Check sheet for the modelled part. Datum: model origin and axes. Units: mm. Give positions to 0.01 mm unless a question says otherwise; leave off trailing zeros. Loops run counter-clockwise (first coordinate to the right, second up) from the corner with the lowest first, then second, coordinate; pieces in that order, holes last. Notation, with made-up numbers: M -31.75,16.5 L -25.75,16.5 A19 ccw -25.75,42.5 Z; hole C 85.5,17 d1. An arc over 180 degrees is marked long. Write each question's results on one line, items separated by ' | '. Start each with the question number.
1. Sectioned sample at B-B on x = 0. Record the cut outline in (y, z) (3 decimals), and give its area (3 significant figures).
2. Go/stop test with a flat-tipped pin: pin 1 (3.5 mm diameter, centred on x = -55.51, z = -55.51, fed in from -Y). Record where the tip stops, or that it passes through.
3. Sectioned sample at C-C on x = -31. Record the cut outline in (y, z).
4. Draft check along Z on faces 1 (the cylindrical face through (-0.65, 1.01, 81.43)), 2 (the cylindrical face through (-51.721, 0.986, -67.453)), 3 (the flat face through (37, 2, 63)). Enter one of: pulls with the +Z half, pulls with the -Z half, needs draft (parallel to the pull), parting line crosses it, or undercut.
5. Material ranges on line 1 along Z through (x, y) = (-0.5, 0.5); line 2 along X through (y, z) = (1.6, -53); line 3 along X through (y, z) = (0.8, -78.5), recorded low to high.
6. Sectioned sample at D-D on y = 1.05. Give the number of separate pieces and of enclosed holes in the cut face, and give its area (3 significant figures).
7. Sectioned sample at A-A on z = 15. Record the cut outline in (x, y).
```python
from build123d import *

# Parameters (mm, degrees)
SKETCH1_R             = 85
SKETCH1_R_2           = 78.5
SKETCH1_R_3           = 72.375
BOSS_EXTRUDE1_DEPTH   = 2
F_6_0MM_DOWEL_HOLE1_D = 6


with BuildPart() as part:
    # Sketch1 → Boss-Extrude1 (new body)
    # profile 1 of 2: a face of its own
    with BuildSketch(Plane(origin=(0, 0, 0), x_dir=(1, 0, 0), z_dir=(0, 1, 0))):
        with Locations(Location((0, 0, 0), (0, 0, 270))):
            Circle(SKETCH1_R)
        Circle(SKETCH1_R_2, mode=Mode.SUBTRACT)
    # profile 2 of 2: a face of its own
    with BuildSketch(Plane(origin=(0, 0, 0), x_dir=(1, 0, 0), z_dir=(0, 1, 0))):
        Circle(SKETCH1_R_2)
        with Locations(Location((0, 0, 0), (0, 0, 270))):
            Circle(SKETCH1_R_3, mode=Mode.SUBTRACT)
    extrude(amount=BOSS_EXTRUDE1_DEPTH)

    # Ø6.0mm Dowel Hole1 (through all)
    with Locations(Plane(origin=(0, 0, 0), x_dir=(-1, 0, 0), z_dir=(0, -1, 0))):
        with Locations((-55.507882323, 55.507882323), (0, 78.5), (55.507882323, 55.507882323), (78.5, 0), (55.507882323, -55.507882323), (0, -78.5), (-55.507882323, -55.507882323), (-78.5, 0)):
            Hole(F_6_0MM_DOWEL_HOLE1_D / 2)


solid = part.part
```
Output values:
1) outline: M 0,-85 L 2,-85 L 2,-81.5 L 0,-81.5 Z; M 0,-75.5 L 2,-75.5 L 2,-72.375 L 0,-72.375 Z; M 0,72.375 L 2,72.375 L 2,75.5 L 0,75.5 Z; M 0,81.5 L 2,81.5 L 2,85 L 0,85 Z | area: 26.5 mm2
2) pin 1: through
3) outline: M 0,-79.15 L 2,-79.15 L 2,-65.4 L 0,-65.4 Z; M 0,65.4 L 2,65.4 L 2,79.15 L 0,79.15 Z
4) face 1: undercut | face 2: parting line crosses it | face 3: needs draft
5) line 1: -85 to -81.46, -75.54 to -72.37, 72.37 to 75.54, 81.46 to 85 | line 2: -66.45 to -57.15, -53.86 to -49.29, 49.29 to 53.86, 57.15 to 66.45 | line 3: -32.6 to -3, 3 to 32.6
6) separate pieces: 1 | enclosed holes: 9 | area: 6,020 mm2
7) outline: M -83.67,0 L -70.8,0 L -70.8,2 L -83.67,2 Z; M 70.8,0 L 83.67,0 L 83.67,2 L 70.8,2 Z
